Here's the drawing with two shaded views (mm, measured from the low corner). I have some questions. Round coordinates to 2 decimals unless told otherwise and drop trailing zeros. Loops run counter-clockwise (first coordinate to the right, second up) from the corner with the lowest first, then second, coordinate; pieces in that order, holes last. Notation, with made-up numbers: M 35,-34 L 62,-34 A29 cw 62,-9 Z; hole C 67,61 d10. An arc over 180 degrees is marked long. Answer as CSV lines item,"result".
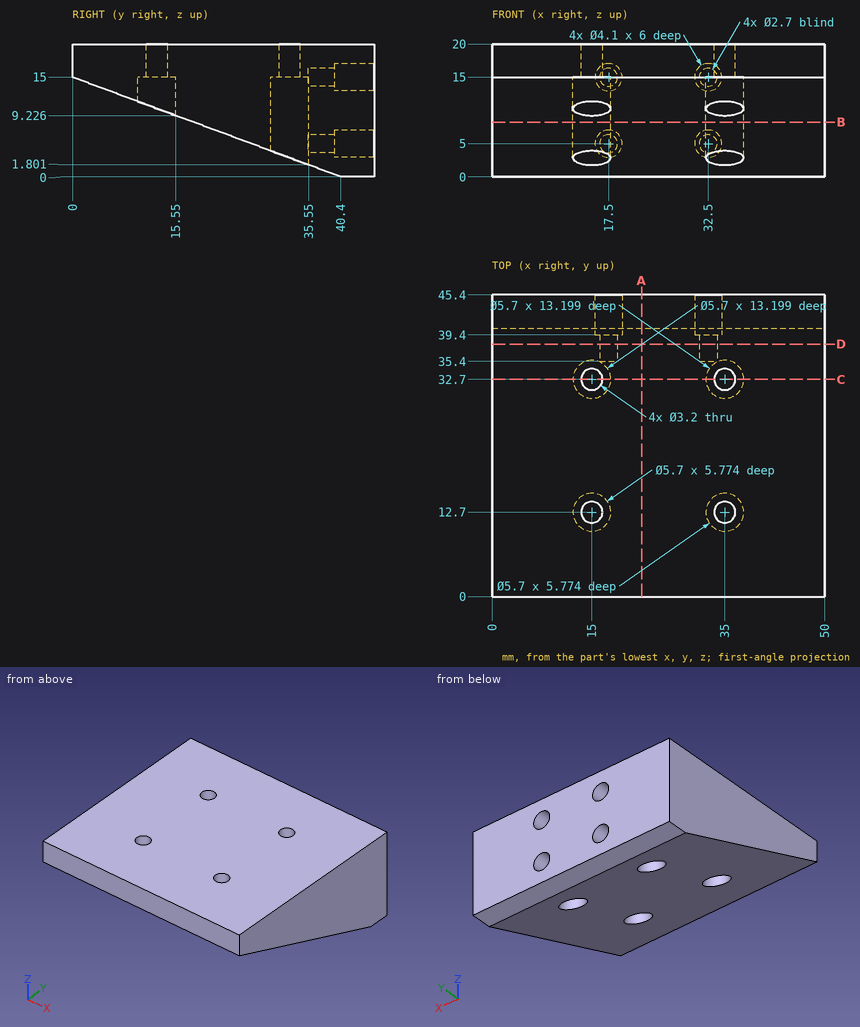
1. I want a section at B-B, the plane z = 8.25. Please give me the cut outline in (x, y).
Evaluation:
outline,"M 0,18.18 L 50,18.18 L 50,45.4 L 0,45.4 Z; hole C 15,32.7 d5.7; hole C 35,32.7 d5.7"
2. For P1, Ø4.5, axis at x = 15, y = 13.5, coming from the -Z side; P2, Ø3, axis at x = 17.5, z = 5.5, coming from the +Y side; P3, Ø3, axis at x = 35.5, y = 33.5, coming from the -Z side, each with a flat end and sliding along its axis, tell me the tip position at first contact or that it passes through.
Evaluation:
P1,"stops at z = 9.15"
P2,"stops at y = 39.4"
P3,"stops at z = 15"
3. I want a section at D-D, the plane y = 38. Please give me the cut outline in (x, z).
Evaluation:
outline,"M 0,0.89 L 50,0.89 L 50,20 L 0,20 Z; hole C 17.5,5 d2.7; hole C 17.5,15 d2.7; hole C 32.5,5 d2.7; hole C 32.5,15 d2.7"
4. I want a section at C-C, the plane y = 32.7. Please give me the cut outline in (x, z).
Evaluation:
outline,"M 0,2.86 L 12.15,2.86 L 12.15,15 L 13.4,15 L 13.4,20 L 0,20 Z; M 16.6,15 L 17.85,15 L 17.85,2.86 L 32.15,2.86 L 32.15,15 L 33.4,15 L 33.4,20 L 16.6,20 Z; M 36.6,15 L 37.85,15 L 37.85,2.86 L 50,2.86 L 50,20 L 36.6,20 Z"
5. If I drill on line 1 (Y direction, x = 35, z = 17.5); line 2 (X direction, y = 43.85, z = 5); line 3 (X direction, y = 36.85, z = 15), over which ranges is the centre line in solid material (lowest first)? Write a range as [from, to].
Evaluation:
line 1,"y = [0, 11.1], [14.3, 31.1], [34.3, 45.4]"
line 2,"x = [0, 15.45], [19.55, 30.45], [34.55, 50]"
line 3,"x = [0, 16.15], [18.85, 31.15], [33.85, 50]"
6. I want a section at A-A, the plane x = 22.5. Please give me the cut outline in (y, z).
Evaluation:
outline,"M 0,15 L 40.4,0 L 45.4,0 L 45.4,20 L 0,20 Z"
